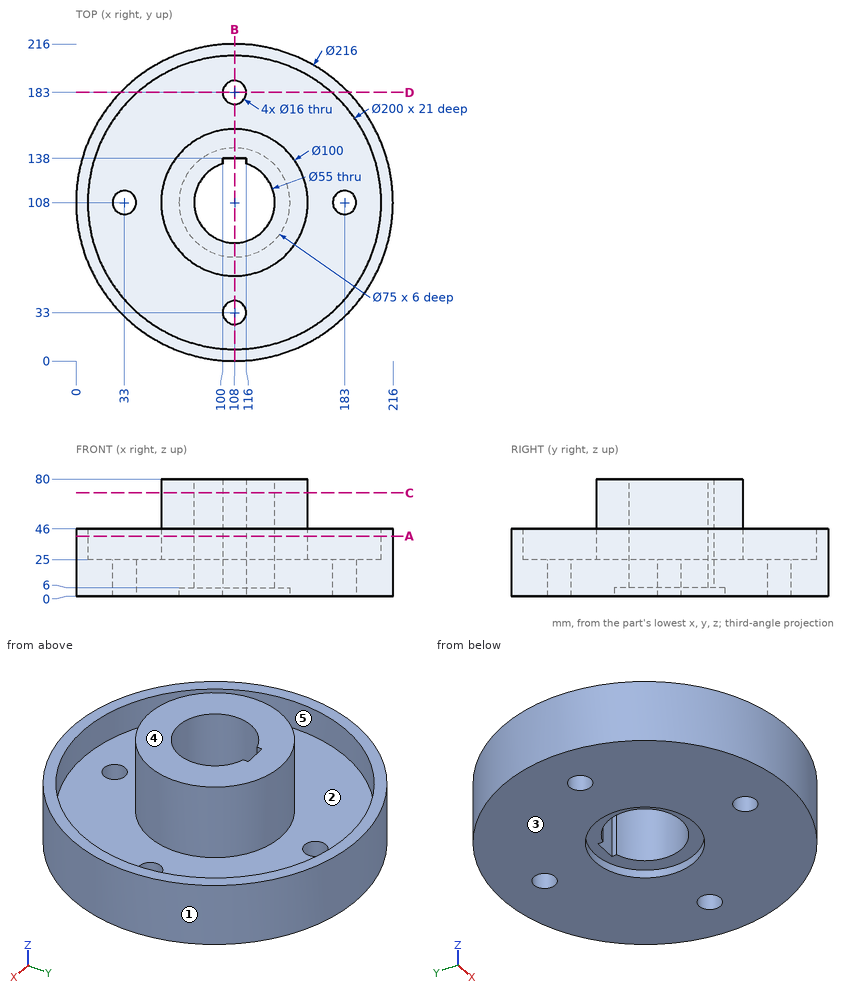
Can you work these out from the drawing? Everything is in mm from the part's minimum corner. A direction names the side the tool comes from. Coordinates: 2 decimals unless noted, no trailing zeros. Write each loop counter-clockwise with the first axis right and the second up, starting at its lowest first coordinate (ties: lowest second). Pieces come first, ordered by that corner, then holes. Notation, with made-up numbers: (5, 78.25) - (43, 78.25) arc R16 ccw to (43, 86.25) - close; hole circle Ø9 at (10, 63). An arc over 180 degrees is marked (long way). One line per item, written item: value.
1) I need wall thicknesses on line 1 along Y through (x, z) = (107, 43) (3 decimals); line 2 along Y through (x, z) = (108, 4); line 3 along Z through (x, y) = (37, 161). Which ranges of each line are inside material? Lowest first, please.
Model answer:
line 1: y = 0.005 to 8.005, 58.01 to 80.518, 138 to 157.99, 207.995 to 215.995
line 2: y = 0 to 25, 41 to 70.5, 145.5 to 175, 191 to 216
line 3: z = 0 to 25
2) Suppose I cut it at C-C on z = 70.5. Write out the boundary of the cut face in (x, y).
Model answer:
outline: circle Ø100 at (108, 108); hole (100, 134.31) arc R27.5 ccw (long way) to (116, 134.31) - (116, 138) - (100, 138) - close
3) We'd pull the mould along Y, two halves only. Please class the marked faces 1, 2 and 3: pulls with the +Y half, pulls with the -Y half, needs draft (parallel to the pull), parting line crosses it, or undercut.
Model answer:
face 1: parting line crosses it
face 2: undercut
face 3: needs draft
4) Suppose I cut it at B-B on x = 108. Write out the boundary of the cut face in (y, z).
Model answer:
outline: (0, 0) - (25, 0) - (25, 25) - (8, 25) - (8, 46) - (0, 46) - close; (41, 0) - (70.5, 0) - (70.5, 6) - (80.5, 6) - (80.5, 80) - (58, 80) - (58, 25) - (41, 25) - close; (138, 6) - (145.5, 6) - (145.5, 0) - (175, 0) - (175, 25) - (158, 25) - (158, 80) - (138, 80) - close; (191, 0) - (216, 0) - (216, 46) - (208, 46) - (208, 25) - (191, 25) - close
5) On a 3-axis mill with a long thin cutter (end or side, diameter ignored), from which of +Z, -Z, +X, -X, +Y, -Y can I reach the whole of each face in a straight line? I mean the marked faces 4 and 5. Say none if no direction works.
Model answer:
face 4: +Z, +X, -X, +Y, -Y
face 5: +Z
6) Suppose I cut it at A-A on z = 41. Write out the boundary of the cut face in (x, y).
Model answer:
outline: circle Ø216 at (108, 108); circle Ø100 at (108, 108); hole circle Ø200 at (108, 108); hole (100, 134.31) arc R27.5 ccw (long way) to (116, 134.31) - (116, 138) - (100, 138) - close
7) Suppose I cut it at D-D on y = 183. Write out the boundary of the cut face in (x, z), and give its area (3 significant figures).
Model answer:
outline: (30.29, 0) - (100, 0) - (100, 25) - (41.86, 25) - (41.86, 46) - (30.29, 46) - close; (116, 0) - (185.71, 0) - (185.71, 46) - (174.14, 46) - (174.14, 25) - (116, 25) - close
area: 3,970 mm²
8) I'm going to push flat-ended pins straight in: P1, Ø1.8, axis at y = 136, z = 60, coming from the +X side; P2, Ø10, axis at x = 150.5, z = 68.5, coming from the +Y side; P3, Ø8, axis at y = 109, z = 47, coming from the +X side; P4, Ø1, axis at x = 42, y = 183, coming from the +Z side. Where does each tip first touch, or does it pass through?
Model answer:
P1: stops at x = 150.02
P2: stops at y = 141.07
P3: stops at x = 216
P4: stops at z = 46
